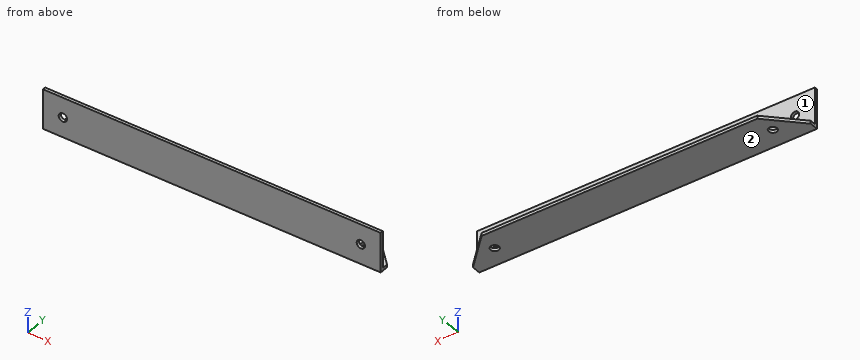
```python
from build123d import *

# Parameters (mm, degrees)
PAD_DEPTH     = 85
SKETCH002_R   = 2.1
HOLE_DEPTH    = 20.001
SKETCH003_R   = 2.1
HOLE001_DEPTH = 20.001
POCKET_DEPTH  = 364.674759


with BuildPart() as part:
    # Sketch → Pad (new body, symmetric)
    with BuildSketch(Plane.YZ):
        Polygon((0, 0), (20, 0), (20, 1.5), (1.5, 1.5), (1.5, 20), (0, 20), align=None)
    extrude(amount=PAD_DEPTH, both=True)

    # Sketch002 → Hole (cut, through all)
    with BuildSketch(Plane.XZ):
        with Locations((-75, 10)):
            Circle(SKETCH002_R)
        with Locations((75, 10)):
            Circle(SKETCH002_R)
    extrude(amount=-HOLE_DEPTH, mode=Mode.SUBTRACT)

    # Sketch003 → Hole001 (cut, through all)
    with BuildSketch(Plane.XY):
        with Locations((-70, 10)):
            Circle(SKETCH003_R)
        with Locations((70, 10)):
            Circle(SKETCH003_R)
    extrude(amount=HOLE001_DEPTH, mode=Mode.SUBTRACT)

    # Sketch004 → Pocket (cut, through all)
    with BuildSketch(Plane.XY):
        Polygon((-85, 4.377634), (-49.377634, 40), (-85, 40), align=None)
    pocket = extrude(amount=POCKET_DEPTH, mode=Mode.SUBTRACT)

    # Mirrored: Pocket across YZ
    add(pocket.mirror(Plane.YZ), mode=Mode.SUBTRACT)


solid = part.part
```
Design review of the part built by this model. Coordinates are the model's own, in mm. Face numbers are marked on the shaded views. A direction names the side the tool comes from. Round coordinates to 2 decimals unless told otherwise and drop trailing zeros. Write each loop counter-clockwise with the first axis right and the second up, starting at its lowest first coordinate (ties: lowest second). Pieces come first, ordered by that corner, then holes.
Item 1: We need section A-A on z = 10. Write out the cut boundary in (x, y).
Item 2: For the marked faces 1 and 2, list the 3-axis set-ups (+Z, -Z, +X, -X, +Y, -Y) from which the entire face can be reached by the end or side of a thin tool; tool diameter is ignored.
Item 3: We need section C-C on x = -75. Write out the cut boundary in (y, z), and give its area (3 significant figures).
Item 4: Clearance check with flat-ended pins moving along their axes: pin 1 Ø2.5 at (x, z) = (-75, 10) entering from -Y; pin 2 Ø3 at (x, z) = (62, 9) entering from +Y; pin 3 Ø2 at (y, z) = (12, 2) entering from +X; pin 4 Ø5.5 at (x, y) = (-25, 11.5) entering from +Z. State where each tip first meets the part, or that it passes through.
Item 5: For probe 1 along Z at (x, y) = (-75, 0.5); probe 2 along X at (y, z) = (10, 0.4); probe 3 along Z at (x, y) = (-36.5, 15.5), list the stretches that pass through material, from the lowest coordinate up.
Item 6: We need section B-B on y = 10. Write out the cut boundary in (x, z), and give its area (3 significant figures).
Item 7: We need section D-D on z = 17.75. Write out the cut boundary in (x, y), and give its area (3 significant figures).
Returned:
1. outline: (-85, 0) - (-77.1, 0) - (-77.1, 1.5) - (-85, 1.5) - close; (-72.9, 0) - (72.9, 0) - (72.9, 1.5) - (-72.9, 1.5) - close; (77.1, 0) - (85, 0) - (85, 1.5) - (77.1, 1.5) - close
2. face 1: +Z, +X, -X, +Y
2. face 2: -Z, +X, -X, +Y, -Y
3. outline: (0, 0) - (14.38, 0) - (14.38, 1.5) - (1.5, 1.5) - (1.5, 7.9) - (0, 7.9) - close; (0, 12.1) - (1.5, 12.1) - (1.5, 20) - (0, 20) - close
3. area: 43.0 mm2
4. pin 1: passes through
4. pin 2: stops at y = 1.5
4. pin 3: stops at x = 78.24
4. pin 4: stops at z = 1.5
5. probe 1: z = 0 to 7.9, 12.1 to 20
5. probe 2: x = -79.38 to -72.1, -67.9 to 67.9, 72.1 to 79.38
5. probe 3: z = 0 to 1.5
6. outline: (-79.38, 0) - (-72.1, 0) - (-72.1, 1.5) - (-79.38, 1.5) - close; (-67.9, 0) - (67.9, 0) - (67.9, 1.5) - (-67.9, 1.5) - close; (72.1, 0) - (79.38, 0) - (79.38, 1.5) - (72.1, 1.5) - close
6. area: 226 mm2
7. outline: (-85, 0) - (85, 0) - (85, 1.5) - (-85, 1.5) - close
7. area: 255 mm2
